Source: CAD feature listing. Evaluate the final solid. Frame: model axes, mm. A direction names the side the tool comes from. Coordinates: 2 decimals unless noted, no trailing zeros. Write each loop counter-clockwise with the first axis right and the second up, starting at its lowest first coordinate (ties: lowest second). Pieces come first, ordered by that corner, then holes. Notation, with made-up numbers: (68.5, -18) -> (77.5, -18) arc R23 cw to (77.5, -7) -> close; hole circle Ø8 at (62.5, -5.5). An arc over 180 degrees is marked (long way). Write item = value, one per line.
from build123d import *

# Parameters (mm, degrees)
EXTRUDE_1_DEPTH              = 8
SKETCH_4_R                   = 2
CUT_EXTRUDE_3_DEPTH          = 31.149626863
HOLE_WIZARD_M4_1_D           = 3.3
HOLE_WIZARD_M4_1_DEPTH       = 10
HOLE_WIZARD_M4_1_CSINK_D     = 4.05
HOLE_WIZARD_M4_1_CSINK_ANGLE = 90
HOLE_WIZARD_M4_1_TIP         = 0.991420021
CHAMFER_1_SIZE               = 0.5


with BuildPart() as part:
    # 草图2 → 凸台-拉伸1 (new body)
    with BuildSketch(Plane.XY):
        Polygon((-7.5, 13), (7.5, 13), (7.5, 10), (26, 10), (26, 0), (-26, 0), (-26, 10), (-7.5, 10), align=None)
    extrude(amount=EXTRUDE_1_DEPTH)

    # 草图4 → 切除-拉伸3 (cut, through all)
    with BuildSketch(Plane.XY.offset(8)):
        with Locations((-22.5, 5)):
            Circle(SKETCH_4_R)
        with Locations(Location((22.5, 5, 0), (0, 0, 180))):
            Circle(SKETCH_4_R)
    extrude(amount=-CUT_EXTRUDE_3_DEPTH, mode=Mode.SUBTRACT)

    # M4 螺纹孔1
    with Locations(Plane(origin=(-15, 10, 4), x_dir=(1, 0, 0), z_dir=(0, 1, 0))):
        with Locations((0, 0), (30, 0)):
            CounterSinkHole(HOLE_WIZARD_M4_1_D / 2, HOLE_WIZARD_M4_1_CSINK_D / 2, depth=HOLE_WIZARD_M4_1_DEPTH, counter_sink_angle=HOLE_WIZARD_M4_1_CSINK_ANGLE)
            with Locations((0, 0, -(HOLE_WIZARD_M4_1_DEPTH + HOLE_WIZARD_M4_1_TIP / 2))):  # 118° drill point
                Cone(0, HOLE_WIZARD_M4_1_D / 2, HOLE_WIZARD_M4_1_TIP, mode=Mode.SUBTRACT)

    # 倒角1
    chamfer_1_edges = [part.edges().sort_by_distance(p)[0] for p in [
        (-7.5, 13, 4),
        (7.5, 13, 4),
    ]]
    chamfer(chamfer_1_edges, length=CHAMFER_1_SIZE)


solid = part.part
1) First-contact query: pin 1 Ø2.5 at (x, z) = (15, 4) entering from +Y; pin 2 Ø0.8 at (y, z) = (11, 3.5) entering from +X; pin 3 Ø0.8 at (y, z) = (10.5, 2.5) entering from -X. Flat tips, straight axial feed; report the tip coordinate or a pass-through.
Answer block:
pin_1 = through
pin_2 = 7.5
pin_3 = -7.5
2) Cut plane D-D, the plane x = 15. Output: boundary loops of the cut face in (y, z) (3 decimals).
Answer block:
outline = (0, 0) -> (10, 0) -> (10, 1.975) -> (9.625, 2.35) -> (0, 2.35) -> close; (0, 5.65) -> (9.625, 5.65) -> (10, 6.025) -> (10, 8) -> (0, 8) -> close
3) Cut plane B-B, the plane x = -22.5. Output: boundary loops of the cut face in (y, z).
Answer block:
outline = (0, 0) -> (3, 0) -> (3, 8) -> (0, 8) -> close; (7, 0) -> (10, 0) -> (10, 8) -> (7, 8) -> close
4) Reachability of faces 4 (the flat face through (17, 10, 6)), 5 (the flat face through (-7.5, 11, 4)), 6 (the flat face through (0, 5, 0)) from +Z, -Z, +X, -X, +Y, -Y: full face, straight path, thin tool, end or side. Return the list, or none.
Answer block:
face_4 = +Z, -Z, +X, +Y
face_5 = +Z, -Z, -X, +Y
face_6 = -Z, +X, -X, +Y, -Y
5) Pull-direction query (X, two-part tool) for faces 1 (the flat face through (7.5, 11, 4)), 2 (the cylindrical face through (13.476, 4.745, 4.632)), 3 (the flat face through (-26, 5, 4)); classes: +X half, -X half, draft (parallel to the pull), parting line (faces both ways), or undercut.
Answer block:
face_1 = +X half
face_2 = undercut
face_3 = -X half
6) Cut plane A-A, the plane y = 5. Output: boundary loops of the cut face in (x, z).
Answer block:
outline = (-26, 0) -> (-24.5, 0) -> (-24.5, 8) -> (-26, 8) -> close; (-20.5, 0) -> (20.5, 0) -> (20.5, 8) -> (-20.5, 8) -> close; (24.5, 0) -> (26, 0) -> (26, 8) -> (24.5, 8) -> close; hole circle Ø3.3 at (-15, 4); hole circle Ø3.3 at (15, 4)
7) Cut plane C-C, the plane z = 4. Output: boundary loops of the cut face in (x, y) (3 decimals).
Answer block:
outline = (-26, 0) -> (-16.65, 0) -> (-16.65, 9.625) -> (-17.025, 10) -> (-26, 10) -> close; (-13.35, 0) -> (13.35, 0) -> (13.35, 9.625) -> (12.975, 10) -> (7.5, 10) -> (7.5, 12.5) -> (7, 13) -> (-7, 13) -> (-7.5, 12.5) -> (-7.5, 10) -> (-12.975, 10) -> (-13.35, 9.625) -> close; (16.65, 0) -> (26, 0) -> (26, 10) -> (17.025, 10) -> (16.65, 9.625) -> close; hole circle Ø4 at (-22.5, 5); hole circle Ø4 at (22.5, 5)
8) Material intervals for probe 1 along Y at (x, z) = (22.5, 3.5); probe 2 along Z at (x, y) = (-15, 7); probe 3 along X at (y, z) = (1.75, 3.5), sorted ascending. Write a range as [from, to].
Answer block:
probe_1 = [0, 3], [7, 10]
probe_2 = [0, 2.35], [5.65, 8]
probe_3 = [-26, -16.57], [-13.43, 13.43], [16.57, 26]
